Part model, mm, in its own coordinate system. Give positions to 0.01 mm unless a question says otherwise; leave off trailing zeros. Loops run counter-clockwise (first coordinate to the right, second up) from the corner with the lowest first, then second, coordinate; pieces in that order, holes last. Notation, with made-up numbers: M 83,68 L 130,68 A22 cw 130,78 Z; hole C 6,-21 d5. An arc over 180 degrees is marked long. Put each result on its own line as item: value. Start each with the question number.
```python
from build123d import *

# Parameters (mm, degrees)
SKETCH1_R           = 330
SKETCH1_R_2         = 82.5
BOSS_EXTRUDE1_DEPTH = 70
SKETCH2_R           = 28.575
CUT_EXTRUDE1_DEPTH  = 131


with BuildPart() as part:
    # Sketch1 → Boss-Extrude1 (new body)
    with BuildSketch(Plane.XY):
        Circle(SKETCH1_R)
        Circle(SKETCH1_R_2, mode=Mode.SUBTRACT)
    extrude(amount=BOSS_EXTRUDE1_DEPTH)

    # Sketch2 → Cut-Extrude1 (cut)
    with BuildSketch(Plane.XY):
        with Locations((0, 290)):
            Circle(SKETCH2_R)
        with Locations((145, 251.147367097)):
            Circle(SKETCH2_R)
        with Locations((251.147367097, 145)):
            Circle(SKETCH2_R)
        with Locations((290, 0)):
            Circle(SKETCH2_R)
        with Locations((251.147367098, -145)):
            Circle(SKETCH2_R)
        with Locations((145, -251.147367097)):
            Circle(SKETCH2_R)
        with Locations((0, -290)):
            Circle(SKETCH2_R)
        with Locations((-145, -251.147367097)):
            Circle(SKETCH2_R)
        with Locations((-251.147367097, -145)):
            Circle(SKETCH2_R)
        with Locations((-290, 0)):
            Circle(SKETCH2_R)
        with Locations((-251.147367097, 145)):
            Circle(SKETCH2_R)
        with Locations((-145, 251.147367097)):
            Circle(SKETCH2_R)
    extrude(amount=CUT_EXTRUDE1_DEPTH, mode=Mode.SUBTRACT)


solid = part.part
```
1) Band-saw the part on A-A on y = 0. Give the cut face in (x, z) (3 decimals).
2) Wall check: L1, parallel to Y at x = 0, z = 32 (3 decimals); L2, parallel to X at y = -145, z = 28; L3, parallel to Y at x = -138, z = 13. Give the ranges that are in metal, low to high.
3) Band-saw the part on D-D on z = 13. State how many separate pieces and enclosed holes the cut face has, then the cut area to 3 significant figures.
4) Pin check, flat tips, straight feed: pin 1 Ø3 at (x, z) = (214, 46) entering from -Y; pin 2 Ø10 at (y, z) = (254.5, 62.5) entering from +X; pin 3 Ø10 at (y, z) = (-59.5, 36) entering from -X. Stop position of each tip, or through.
5) Band-saw the part on C-C on x = -165. Give the cut face in (y, z).
6) Band-saw the part on B-B on y = 290. Give the cut face in (x, z) (3 decimals).
Evaluation:
1. outline: M -330,0 L -318.575,0 L -318.575,70 L -330,70 Z; M -261.425,0 L -82.5,0 L -82.5,70 L -261.425,70 Z; M 82.5,0 L 261.425,0 L 261.425,70 L 82.5,70 Z; M 318.575,0 L 330,0 L 330,70 L 318.575,70 Z
2. L1: -330 to -318.575, -261.425 to -82.5, 82.5 to 261.425, 318.575 to 330
2. L2: -296.44 to -279.72, -222.57 to 222.57, 279.72 to 296.44
2. L3: -299.76 to -278.85, -223.44 to 223.44, 278.85 to 299.76
3. separate pieces: 1
3. enclosed holes: 13
3. area: 290,000 mm2
4. pin 1: y = -252.48
4. pin 2: x = 215.99
4. pin 3: x = -325.47
5. outline: M -285.79,0 L -271.56,0 L -271.56,70 L -285.79,70 Z; M -230.74,0 L 230.74,0 L 230.74,70 L -230.74,70 Z; M 271.56,0 L 285.79,0 L 285.79,70 L 271.56,70 Z
6. outline: M -157.48,0 L -28.575,0 L -28.575,70 L -157.48,70 Z; M 28.575,0 L 157.48,0 L 157.48,70 L 28.575,70 Z
